```python
from build123d import *

# Parameters (mm, degrees)
SKETCH1_W                  = 60
SKETCH1_H                  = 46
BOSS_EXTRUDE1_DEPTH        = 7.55
FILLET1_R                  = 10
F_8_0_8_DIAMETER_HOLE1_D   = 8
SKETCH4_W                  = 60
SKETCH4_H                  = 10
BOSS_EXTRUDE2_DEPTH        = 64
CUT_EXTRUDE1_DEPTH         = 50
SKETCH7_4_R                = 17
BOSS_EXTRUDE3_DEPTH        = 44.58869
SKETCH11_W                 = 10
SKETCH11_H                 = 10
BOSS_EXTRUDE4_DEPTH        = 40
F_18_0_18_DIAMETER_HOLE1_D = 18


with BuildPart() as part:
    # Sketch1 → Boss-Extrude1 (new body)
    with BuildSketch(Plane(origin=(0, 0, 0), x_dir=(1, 0, 0), z_dir=(0, 1, 0))):
        with Locations((30, 23)):
            Rectangle(SKETCH1_W, SKETCH1_H)
    extrude(amount=BOSS_EXTRUDE1_DEPTH)

    # Fillet1
    fillet1_edges = [part.edges().sort_by_distance(p)[0] for p in [
        (0, 3.775, -46),
        (60, 3.775, -46),
        (60, 3.775, 0),
        (0, 3.775, 0),
    ]]
    fillet(fillet1_edges, radius=FILLET1_R)

    # Ø8.0 (8) Diameter Hole1 (through all)
    with Locations(Plane(origin=(50, 7.55, -10), x_dir=(0, 0, 1), z_dir=(0, 1, 0))):
        with Locations((0, 0), (0, -40), (-26, -40), (-26, 0)):
            Hole(F_8_0_8_DIAMETER_HOLE1_D / 2)

    # Sketch4 → Boss-Extrude2 (add, along a direction that is not the sketch's normal)
    with BuildSketch(Plane(origin=(0, 7.55, 0), x_dir=(1, 0, 0), z_dir=(0, 1, 0))):
        with Locations((30, 23)):
            Rectangle(SKETCH4_W, SKETCH4_H)
    extrude(amount=BOSS_EXTRUDE2_DEPTH, dir=(-0.6691306063588565, 0.7431448254773959, 0))

    # Sketch7 → Cut-Extrude1 (cut)
    with BuildSketch(Plane(origin=(36.890174053, 33.216061912, 0), x_dir=(0, 0, -1), z_dir=(0.7431448254773956, 0.6691306063588568, 0))):
        with BuildLine():
            Line((14.444935509, 45.97411464), (14.444935509, 31.283611873))
            Line((14.444935509, 31.283611873), (33.990304022, 31.283611873))
            Line((33.990304022, 31.283611873), (33.990304022, 44.253315706))
            ThreePointArc((33.990304022, 44.253315706), (24.490934317, 48.218106695), (14.444935509, 45.97411464))
        make_face()
    extrude(amount=-CUT_EXTRUDE1_DEPTH, mode=Mode.SUBTRACT)


with BuildPart() as cut_extrude1_kept_piece:
    # of the separate pieces the step leaves, the one the design keeps (cut_extrude1_pieces_kept)
    add(part.part.solids().sort_by_distance((10, 0, 0))[0])

    # Sketch7<4> → Boss-Extrude3 (add)
    with BuildSketch(Plane(origin=(36.890174053, 33.216061912, 0), x_dir=(0, 0, -1), z_dir=(0.7431448254773956, 0.6691306063588568, 0))):
        with Locations((23, 31.283611873)):
            Circle(SKETCH7_4_R)
    extrude(amount=-BOSS_EXTRUDE3_DEPTH)

    # Sketch11 → Boss-Extrude4 (add, along a direction that is not the sketch's normal)
    with BuildSketch(Plane(origin=(0, 7.55, 0), x_dir=(1, 0, 0), z_dir=(0, 1, 0))):
        with Locations((30, 33)):
            Rectangle(SKETCH11_W, SKETCH11_H)
        with Locations((30, 13)):
            Rectangle(SKETCH11_W, SKETCH11_H)
    extrude(amount=BOSS_EXTRUDE4_DEPTH, dir=(-0.6691306063588565, 0.7431448254773958, 0))

    # Ø18.0 (18) Diameter Hole1 (through all)
    with Locations(Plane(origin=(15.957351871, 56.464316198, -23), x_dir=(-0.669130606359, 0.743144825477, 0), z_dir=(0.743144825477, 0.669130606359, 0))):
        with Locations((0, 0)):
            Hole(F_18_0_18_DIAMETER_HOLE1_D / 2)


solid = cut_extrude1_kept_piece.part
```
Work out the finished part from the listing and answer in its coordinate system (mm). A direction names the side the tool comes from. Give positions to 0.01 mm unless a question says otherwise; leave off trailing zeros. Loops run counter-clockwise (first coordinate to the right, second up) from the corner with the lowest first, then second, coordinate; pieces in that order, holes last. Notation, with made-up numbers: M 74.5,83 L 118.5,83 A22 ccw 118.5,105 Z; hole C 38.5,-26 d4. An arc over 180 degrees is marked long. One line per item, written item: value. Start each with the question number.
1. Each of these flat-tipped pins is pushed along its axis until it touches: P1, Ø4, axis at y = 4.5, z = -21, coming from the -X side; P2, Ø8, axis at y = 30, z = -35, coming from the +X side; P3, Ø1.5, axis at x = -18.5, z = -12.5, coming from the +Y side; P4, Ø12, axis at x = -16.5, y = 11, coming from the +Z side. Where does it stop, or does it pass through?
2. Find the intervals of material crossed by probe 1 along X at (y, z) = (4.25, -36); probe 2 along Y at (x, z) = (14.5, -8.5); probe 3 along Z at (x, y) = (-2, 51.5), in increasing order.
3. Find section A-A (z = -15). Give the vertices of the cut face in (x, y).
4. Find section C-C (x = 44.5). Give the vertices of the cut face in (y, z).
5. Which of the six approach directions +Z, -Z, +X, -X, +Y, -Y give full straight-line access (tool end or side, diameter ignored) to faces 4 (the face through (21.805, 22.205, -12.93)), 5 (the face through (2.85, 3.83, -3.01)), 6 (the face through (9, 15, -18))?
6. Find section B-B (x = 33). Give the vertices of the cut face in (y, z).
7. Determine the mould class of faces 1 (the face through (36, 22, -18)), 2 (the face through (25.75, 45.59, -22.76)), 3 (the face through (57.15, 3.83, -42.99)) for opening direction Y: released by +Y, released by -Y, zero draft, split by the parting line, or undercut.
Reported:
1. P1: stops at x = 0
1. P2: stops at x = 18.39
1. P3: stops at y = 44.45
1. P4: passes through
2. probe 1: x = 0 to 6, 14 to 46, 54 to 60
2. probe 2: y = 0 to 7.55, 19.21 to 30.32, 43.21 to 58.08
2. probe 3: z = -37.82 to -26.42, -19.58 to -8.18
3. outline: M -27.22,37.78 L -19.94,29.69 L 13.2,59.53 L 5.92,67.61 Z; M -14.42,23.56 L -7.14,15.48 L 6.67,27.91 L 25,7.55 L 0,7.55 L 0,0 L 60,0 L 60,7.55 L 35,7.55 L 12.19,32.89 L 25.99,45.32 L 18.72,53.4 Z
4. outline: M 0,-46 L 7.55,-46 L 7.55,-28 L 24.76,-28 L 24.76,-18 L 7.55,-18 L 7.55,0 L 0,0 Z
5. face 4: +Z, +X
5. face 5: +Z, -X, -Y
5. face 6: +Z
6. outline: M 0,-46 L 7.55,-46 L 7.55,-38 L 9.77,-38 L 9.77,-28 L 37.54,-28 L 37.54,-18 L 9.77,-18 L 9.77,-8 L 7.55,-8 L 7.55,0 L 0,0 Z
7. face 1: undercut
7. face 2: released by +Y
7. face 3: zero draft
